Geometry: see drawing. Coordinates: mm, zero at the bounding-box minimum. A direction names the side the tool comes from. Give positions to 0.01 mm unless a question says otherwise; leave off trailing zeros. Write each loop counter-clockwise with the first axis right and the second up, starting at its lowest first coordinate (ties: lowest second). Pieces come first, ordered by that corner, then holes.
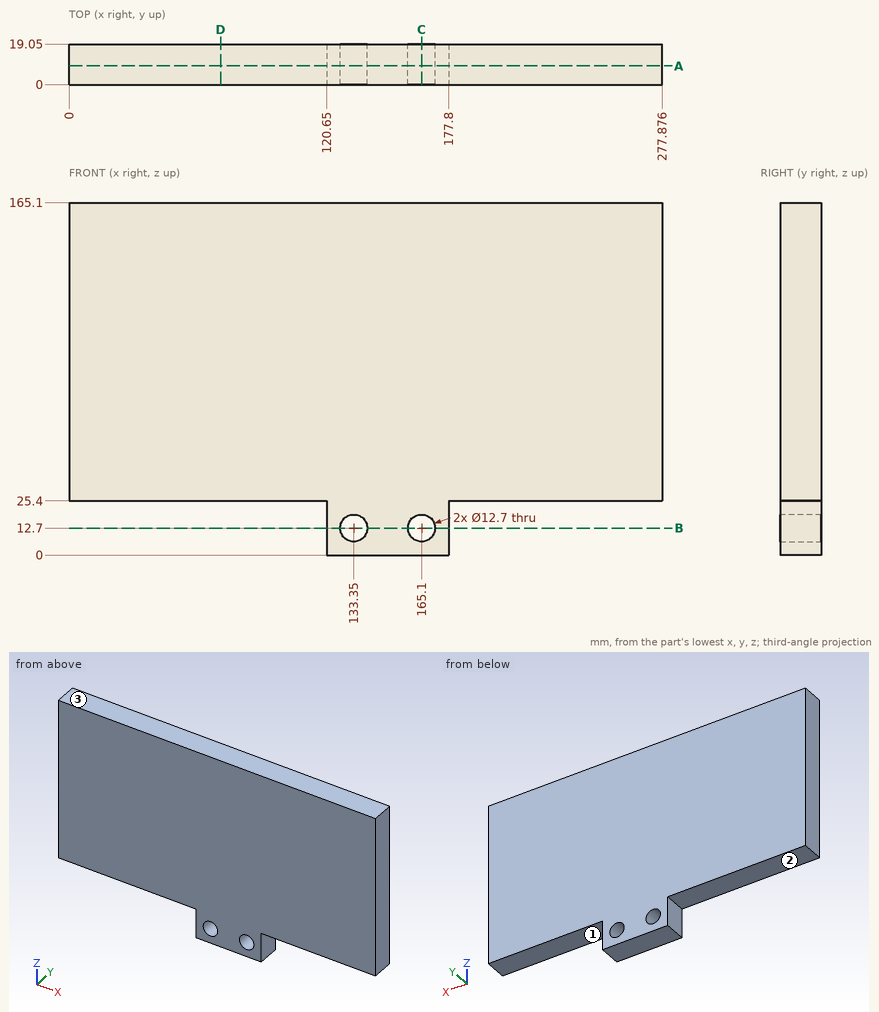
1. Section query D-D (x = 71). Return loops of the section in (y, z).
2. Section query A-A (y = 8.75). Return loops of the section in (x, z), plus the area to 3 significant figures.
3. Access query for the marked faces 1, 2 and 3. Directions: +Z, -Z, +X, -X, +Y, -Y. A direction counts if a zero-diameter tool reaches every point of the face in a straight line with its end or side. Return the directions, or none.
4. Line query: probe 1 along X at (y, z) = (10.5, 12.7); probe 2 along X at (y, z) = (17.25, 23); probe 3 along Z at (x, y) = (42, 1.25). Output: solid intervals per line, ascending.
5. Section query C-C (x = 165.1). Return loops of the section in (y, z), plus the area to 3 significant figures.
6. Pin query (flat end, axial travel): P1, Ø5.5, axis at x = 55.5, y = 8.5, coming from the -Z side. Return the tip coordinate at first contact, or that it passes through.
7. Section query B-B (z = 12.7). Return loops of the section in (x, y).
The answers:
1. outline: (0, 25.4) - (19.05, 25.4) - (19.05, 165.1) - (0, 165.1) - close
2. outline: (0, 25.4) - (120.65, 25.4) - (120.65, 0) - (177.8, 0) - (177.8, 25.4) - (277.88, 25.4) - (277.88, 165.1) - (0, 165.1) - close; hole circle Ø12.7 at (133.35, 12.7); hole circle Ø12.7 at (165.1, 12.7)
2. area: 40,000 mm2
3. face 1: -Z, +X, +Y, -Y
3. face 2: -Z, -X, +Y, -Y
3. face 3: +Z, +X, -X, +Y, -Y
4. probe 1: x = 120.65 to 127, 139.7 to 158.75, 171.45 to 177.8
4. probe 2: x = 120.65 to 177.8
4. probe 3: z = 25.4 to 165.1
5. outline: (0, 0) - (19.05, 0) - (19.05, 6.35) - (0, 6.35) - close; (0, 19.05) - (19.05, 19.05) - (19.05, 165.1) - (0, 165.1) - close
5. area: 2,900 mm2
6. P1: stops at z = 25.4
7. outline: (120.65, 0) - (127, 0) - (127, 19.05) - (120.65, 19.05) - close; (139.7, 0) - (158.75, 0) - (158.75, 19.05) - (139.7, 19.05) - close; (171.45, 0) - (177.8, 0) - (177.8, 19.05) - (171.45, 19.05) - close
